The model under review builds one solid part; all positions refer to its coordinate system, in mm. A direction names the side the tool comes from. Coordinates: 2 decimals unless noted, no trailing zeros. Write each loop counter-clockwise with the first axis right and the second up, starting at its lowest first coordinate (ties: lowest second). Pieces come first, ordered by that corner, then holes. Notation, with made-up numbers: (62, 16.25) - (70, 16.25) arc R27 ccw to (70, 32.25) - close; hole circle Ø10 at (59.5, 10.5). An arc over 180 degrees is marked (long way). Put each result on its own line as item: value. Start each with the question number.
Item 1: Consider section B-B on x = -2.5. Give the boundary of the cut face in (y, z), then the cut area to 3 significant figures.
Item 2: To check wall thickness, follow L1, parallel to Z at x = -16, y = -5.25; L2, parallel to Z at x = 8.5, y = -1.75; L3, parallel to Z at x = -4, y = -6.75. State the ranges of each line that lie inside material, in increasing order. Write a range as [from, to].
Item 3: Mouldability with a two-part tool opening along Z and no side actions: class faces 3 (the face through (-20, -5, 0)), 4 (the face through (17.583, -4.93, -7.2)), 5 (the face through (-19, -5, 18)), 6 (the face through (19, -5, -18)) as pulls with the +Z half, pulls with the -Z half, needs draft (parallel to the pull), parting line crosses it, or undercut.
Item 4: Machinability: for faces 1 (the face through (-7.88, -4.93, -10.71)), 2 (the face through (0, -5, 20)), which of the approach directions +Z, -Z, +X, -X, +Y, -Y give a long, thin tool a straight path to every point of the face, cutting with its end or side? Answer none if there is none.
Item 5: Consider section D-D on y = -8.5. State how many separate pieces and enclosed holes the cut face has, then the cut area to 3 significant figures.
Item 6: Consider section A-A on z = -16. Give the boundary of the cut face in (x, y), then the cut area to 3 significant figures.
Item 7: For pin 1 (3 mm diameter, centred on x = 16, z = 16, fed in from +Y), flat-tipped, find the tip position at first contact; note if it passes through.
Item 8: Consider section C-C on x = -16. Give the boundary of the cut face in (y, z).
Solid Edge part; units mm, degrees
sketch "Sketch1" plane through (0, 0, 0) normal (0, -1, 0) x (1, 0, 0)
  circle A0 centre (16, 16) radius 2
  circle A1 centre (-16, 16) radius 2
  circle A2 centre (-16, -16) radius 2
  circle A3 centre (16, -16) radius 2
  line L0 (-2, -7.2284) -> (-2, -18.8944)
  arc A4 (-2, -18.8944) -> (-11.9462, -14.7746) centre (0, 0) cw
  line L1 (-11.9462, -14.7746) -> (-3.697, -6.5255)
  arc A5 (-2, -7.2284) -> (-3.697, -6.5255) centre (0, 0) cw
  arc A6 (18.8944, -2) -> (14.7746, -11.9462) centre (0, 0) cw
  line L2 (14.7746, -11.9462) -> (6.5255, -3.697)
  line L3 (7.2284, -2) -> (18.8944, -2)
  arc A7 (6.5255, -3.697) -> (7.2284, -2) centre (0, 0) ccw
  line L4 (-14.7746, 11.9462) -> (-6.5255, 3.697)
  arc A8 (-7.2284, 2) -> (-6.5255, 3.697) centre (0, 0) cw
  line L5 (-7.2284, 2) -> (-18.8944, 2)
  arc A9 (-18.8944, 2) -> (-14.7746, 11.9462) centre (0, 0) cw
  line L6 (-2, 18.8944) -> (-2, 7.2284)
  arc A10 (-3.697, 6.5255) -> (-2, 7.2284) centre (0, 0) cw
  line L7 (-3.697, 6.5255) -> (-11.9462, 14.7746)
  arc A11 (-11.9462, 14.7746) -> (-2, 18.8944) centre (0, 0) cw
  arc A12 (-6.5255, -3.697) -> (-7.2284, -2) centre (0, 0) cw
  line L8 (-18.8944, -2) -> (-7.2284, -2)
  arc A13 (-14.7746, -11.9462) -> (-18.8944, -2) centre (0, 0) cw
  line L9 (-6.5255, -3.697) -> (-14.7746, -11.9462)
  line L10 (2, 7.2284) -> (2, 18.8944)
  arc A14 (2, 18.8944) -> (11.9462, 14.7746) centre (0, 0) cw
  line L11 (11.9462, 14.7746) -> (3.697, 6.5255)
  arc A15 (2, 7.2284) -> (3.697, 6.5255) centre (0, 0) cw
  line L12 (2, -18.8944) -> (2, -7.2284)
  arc A16 (3.697, -6.5255) -> (2, -7.2284) centre (0, 0) cw
  line L13 (3.697, -6.5255) -> (11.9462, -14.7746)
  arc A17 (11.9462, -14.7746) -> (2, -18.8944) centre (0, 0) cw
  line L14 (18.8944, 2) -> (7.2284, 2)
  arc A18 (6.5255, 3.697) -> (7.2284, 2) centre (0, 0) cw
  line L15 (6.5255, 3.697) -> (14.7746, 11.9462)
  arc A19 (14.7746, 11.9462) -> (18.8944, 2) centre (0, 0) cw
  line L16 (-15, -20) -> (15, -20)
  arc A20 (20, -15) -> (15, -20) centre (15, -15) cw
  line L17 (20, -15) -> (20, 15)
  arc A21 (15, 20) -> (20, 15) centre (15, 15) cw
  line L18 (15, 20) -> (-15, 20)
  arc A22 (-20, 15) -> (-15, 20) centre (-15, 15) cw
  line L19 (-20, 15) -> (-20, -15)
  arc A23 (-20, -15) -> (-15, -20) centre (-15, -15) ccw
extrude "Protrusion1" add sketch "Sketch1" along normal blind 10
Report:
1. outline: (-10, -20) - (0, -20) - (0, -18.83) - (-10, -18.83) - close; (-10, -7.07) - (0, -7.07) - (0, 7.07) - (-10, 7.07) - close; (-10, 18.83) - (0, 18.83) - (0, 20) - (-10, 20) - close
1. area: 165 mm²
2. L1: [-19.9, -18], [-14, -10.25], [-2, 2], [10.25, 14], [18, 19.9]
2. L2: [-20, -16.99], [-11.33, -5.67], [-2, 2], [5.67, 11.33], [16.99, 20]
2. L3: [-20, -18.57], [-6.83, 6.83], [18.57, 20]
3. face 3: needs draft
3. face 4: undercut
3. face 5: pulls with the +Z half
3. face 6: pulls with the -Z half
4. face 1: +Y, -Y
4. face 2: +Z, +X, -X, +Y, -Y
5. separate pieces: 1
5. enclosed holes: 12
5. area: 941 mm²
6. outline: (-19.9, -10) - (-18, -10) - (-18, 0) - (-19.9, 0) - close; (-14, -10) - (-10.25, -10) - (-10.25, 0) - (-14, 0) - close; (-2, -10) - (2, -10) - (2, 0) - (-2, 0) - close; (10.25, -10) - (14, -10) - (14, 0) - (10.25, 0) - close; (18, -10) - (19.9, -10) - (19.9, 0) - (18, 0) - close
6. area: 153 mm²
7. pin 1: through
8. outline: (-10, -19.9) - (0, -19.9) - (0, -18) - (-10, -18) - close; (-10, -14) - (0, -14) - (0, -10.25) - (-10, -10.25) - close; (-10, -2) - (0, -2) - (0, 2) - (-10, 2) - close; (-10, 10.25) - (0, 10.25) - (0, 14) - (-10, 14) - close; (-10, 18) - (0, 18) - (0, 19.9) - (-10, 19.9) - close
